Model file for the job. Use its own axes, mm. A direction names the side the tool comes from. Coordinates: 2 decimals unless noted, no trailing zeros. Order: outer loops, then holes, each group sorted by start corner. A loop starts at its lowest first (then second) coordinate and runs counter-clockwise, first axis right, second up. Notation, with made-up numbers: M -16.5,69 L 23.5,69 A24 cw 23.5,97 Z; hole C 40.25,-19.75 d4. An arc over 180 degrees is marked long. Return JSON: item names as keys, results as strings.
Autodesk Inventor part; units mm, degrees
ref_plane "Work Plane1" through (-101.6, 10.414, 26.858) normal (0, 0, 1) x (1, 0, 0)
ref_plane "Work Plane2" through (101.6, 10.414, -26.858) normal (0, 0, -1) x (-1, 0, 0)
ref_plane "YZ Plane" through (0, 0, 0) normal (1, 0, 0) x (0, 1, 0)
sketch "Sketch1" plane through (0, 0, 0) normal (1, 0, 0) x (0, 1, 0)
  line L0 (-19.05, 6.858) -> (19.05, 6.858)
  line L1 (19.05, 6.858) -> (19.05, -6.858)
  line L2 (19.05, -6.858) -> (-19.05, -6.858)
  line L3 (-19.05, -6.858) -> (-19.05, 6.858)
  line L4 (-19.05, 6.858) -> (19.05, -6.858) construction
  line L5 (19.05, 6.858) -> (-19.05, -6.858) construction
  arc A0 (19.05, 6.858) -> (10.414, 6.858) centre (14.732, 4.0649) ccw
  arc A1 (10.414, -6.858) -> (19.05, -6.858) centre (14.732, -4.0649) ccw
  line L6 (14.732, 9.2075) -> (14.732, -9.2075)
  point P0 (0, 0)
  dimension "d0" = 38.1
  dimension "d1" = 13.716
  dimension "d6" = 8.636
  dimension "d8" = 8.636
  dimension "d9" = 18.415
extrude "Extrusion1" add sketch "Sketch1" along normal mid plane 203.2
sketch "Sketch3" plane through (-101.6, -19.05, -6.858) normal (0, -1, 0) x (1, 0, 0)
  line L0 (0, 0) -> (203.2, 0)
  line L1 (203.2, 13.716) -> (203.2, 0)
  line L2 (203.2, 13.716) -> (0, 13.716)
  line L3 (0, 0) -> (0, 13.716)
  line L4 (203.2, 6.858) -> (154.94, 6.858)
  line L5 (154.94, 6.858) -> (154.94, 3.8)
  line L6 (154.94, 3.8) -> (203.2, 3.8)
  line L7 (203.2, 3.8) -> (203.2, 6.858)
  line L8 (154.94, 6.858) -> (203.2, 6.858)
  line L9 (203.2, 6.858) -> (203.2, 9.916)
  line L10 (0, 9.916) -> (48.26, 9.916)
  line L11 (48.26, 9.916) -> (48.26, 6.858)
  line L12 (48.26, 6.858) -> (0, 6.858)
  line L13 (0, 6.858) -> (0, 9.916)
  point P0 (101.6, 6.858)
  dimension "d14" = 48.26
  dimension "d19" = 3.8
  dimension "d21" = 3.058
  dimension "d22" = 48.26
  dimension "d23" = 3.8
  dimension "d24" = 3.058
extrude "Extrusion3" cut sketch "Sketch3" against normal through all contours L3 L10 L11 L12 | L6 L5 L4 L1
ref_plane "Work Plane1" through (-101.6, 10.414, 26.858) normal (0, 0, 1) x (1, 0, 0)
sketch "Sketch4" plane through (-101.6, 10.414, 26.858) normal (0, 0, 1) x (1, 0, 0)
  line L0 (0, 0) -> (203.2, 0)
  line L1 (0, -29.464) -> (0, 0)
  line L2 (203.2, -29.464) -> (0, -29.464)
  line L3 (203.2, 0) -> (203.2, -29.464)
  line L4 (0, 0) -> (203.2, 0)
  line L5 (203.2, 8.636) -> (203.2, 0)
  line L6 (0, 8.636) -> (203.2, 8.636)
  line L7 (0, 0) -> (0, 8.636)
  line L8 (203.2, 8.636) -> (165.1, -29.464)
  line L9 (0, 8.636) -> (38.1, -29.464)
  line L10 (203.2, 8.636) -> (203.2, -29.464)
  line L11 (165.1, -29.464) -> (203.2, -29.464)
  line L12 (38.1, -29.464) -> (0, -29.464)
  line L13 (0, 8.636) -> (0, -29.464)
  point P0 (101.6, -10.414)
  dimension "d28" = 45
  dimension "d29" = 45
extrude "Extrusion4" cut sketch "Sketch4" against normal blind 23.8 contours L7 L9 L0 | L0 L9 L2 L1 | L8 L5 L0 | L0 L3 L2 L8
ref_plane "Work Plane2" through (101.6, 10.414, -26.858) normal (0, 0, -1) x (-1, 0, 0)
sketch "Sketch5" plane through (101.6, 10.414, -26.858) normal (0, 0, -1) x (-1, 0, 0)
  line L0 (203.2, 0) -> (0, 0)
  line L1 (0, -29.464) -> (0, 0)
  line L2 (203.2, -29.464) -> (0, -29.464)
  line L3 (203.2, 0) -> (203.2, -29.464)
  line L4 (0, 8.636) -> (203.2, 8.636)
  line L5 (0, 0) -> (0, 8.636)
  line L6 (203.2, 0) -> (0, 0)
  line L7 (203.2, 8.636) -> (203.2, 0)
  line L8 (0, 8.636) -> (38.1, -29.464)
  line L9 (203.2, 8.636) -> (165.1, -29.464)
  line L10 (165.1, -29.464) -> (203.2, -29.464)
  line L11 (203.2, -29.464) -> (203.2, 8.636)
  line L12 (38.1, -29.464) -> (0, -29.464)
  line L13 (0, -29.464) -> (0, 8.636)
  point P0 (101.6, -10.414)
  dimension "d33" = 45
  dimension "d34" = 45
extrude "Extrusion5" cut sketch "Sketch5" against normal blind 23.8 contours L3 L2 L9 L0 | L0 L9 L7 | L8 L2 L1 L0 | L0 L5 L8
equation "\"d14\" = SlotDepth"
equation "\"d19\" = SlotOffset"
equation "\"d21\" = SlotWidth"
equation "\"d22\" = SlotDepth"
equation "\"d23\" = SlotOffset"
equation "\"d24\" = SlotWidth"
equation "\"d0\" = StretcherHeight"
equation "\"d1\" = StretcherDepth"
equation "\"d6\" = RoundoverDiameter"
equation "\"d8\" = d6"
properties part number "Stretcher-08" material "Wood (Birch)"
Item 1: Drop flat-ended pins along their axis: pin 1 Ø14.5 at (x, y) = (-17.5, -7.5) entering from -Z; pin 2 Ø3 at (y, z) = (7, -4) entering from +X; pin 3 Ø19 at (x, y) = (66, 0) entering from +Z. Give the stop position or say it passes through.
Check result:
{"pin 1": "stops at z = -6.86", "pin 2": "stops at x = 91.05", "pin 3": "stops at z = 6.86"}
Item 2: Saw through at A-A (x = -59). Write the cut outline in (y, z).
Check result:
{"outline": "M -19.05,-6.86 L 10.41,-6.86 A5.14 ccw 19.05,-6.86 L 19.05,0 L -19.05,0 Z; M -19.05,3.06 L 19.05,3.06 L 19.05,6.86 A5.14 ccw 10.41,6.86 L -19.05,6.86 Z"}
Item 3: Saw through at D-D (x = 34). Write the cut outline in (y, z).
Check result:
{"outline": "M -19.05,-6.86 L 10.41,-6.86 A5.14 ccw 19.05,-6.86 L 19.05,6.86 A5.14 ccw 10.41,6.86 L -19.05,6.86 Z"}
Item 4: Wall check: line 1 (Z direction, x = 55.5, y = -15.5); line 2 (Z direction, x = 51.5, y = -10.5); line 3 (X direction, y = 11, z = 2.5). Give the ranges that are in metal, low to high.
Check result:
{"line 1": "z = -6.86 to -3.06, 0 to 6.86", "line 2": "z = -6.86 to 6.86", "line 3": "x = -53.34 to 101.6"}
Item 5: 3-axis set-ups, long thin cutter, end or side, ignore diameter. For faces 1 (the flat face through (82.82, 0.27, -4.81)), 2 (the flat face through (-1, -5, 6.858)), 3 (the flat face through (-91, -8, -3.058)), 4 (the flat face through (72, 4, -3.058)), 5 (the flat face through (-82.82, 0.27, 4.81)): which of +Z, -Z, +X, -X, +Y, -Y reach the whole face in a straight line?
Check result:
{"face 1": "-Z, +X, -Y", "face 2": "+Z, +X, -X, -Y", "face 3": "-Z, -X, -Y", "face 4": "+X, +Y, -Y", "face 5": "+Z, -X, -Y"}
Item 6: Pull direction Z, two halves, no side cores. Call faces 6 (the flat face through (-77, 0, 0)), 7 (the flat face through (91, -8, 3.058)), 8 (the flat face through (-1, -4, -6.858)), 9 (the flat face through (-82.82, 0.27, -4.81)): +Z half, -Z half, draft (parallel to the pull), parting line (faces both ways), or undercut.
Check result:
{"face 6": "undercut", "face 7": "+Z half", "face 8": "-Z half", "face 9": "draft"}
Item 7: Saw through at B-B (y = 2). Write the cut outline in (x, z).
Check result:
{"outline": "M -101.6,-3.06 L -84.55,-3.06 L -84.55,-6.86 L 84.55,-6.86 L 84.55,-3.06 L 53.34,-3.06 L 53.34,0 L 101.6,0 L 101.6,3.06 L 84.55,3.06 L 84.55,6.86 L -84.55,6.86 L -84.55,3.06 L -53.34,3.06 L -53.34,0 L -101.6,0 Z"}
Item 8: Saw through at C-C (x = -82.5). Write the cut outline in (y, z), and give its area (3 significant figures).
Check result:
{"outline": "M -19.05,-3.06 L -0.05,-3.06 L -0.05,-6.86 L 10.41,-6.86 A5.14 ccw 19.05,-6.86 L 19.05,0 L -19.05,0 Z; M -0.05,3.06 L 19.05,3.06 L 19.05,6.86 A5.14 ccw 10.41,6.86 L -0.05,6.86 Z", "area": "290 mm2"}
